The figure shows three views and two pictorial views of one solid part (mm, origin at its lowest corner). Answer the questions. A direction names the side the tool comes from. Round coordinates to 2 decimals unless told otherwise and drop trailing zeros. Order: outer loops, then holes, each group sorted by start corner. A loop starts at its lowest first (then second) coordinate and runs counter-clockwise, first axis right, second up. Notation, with made-up numbers: M 14.25,85.5 L 21.25,85.5 A23 ccw 21.25,110.5 Z; hole C -2,39 d5. An arc over 180 degrees is marked long. Return JSON: item names as keys, results as strings.
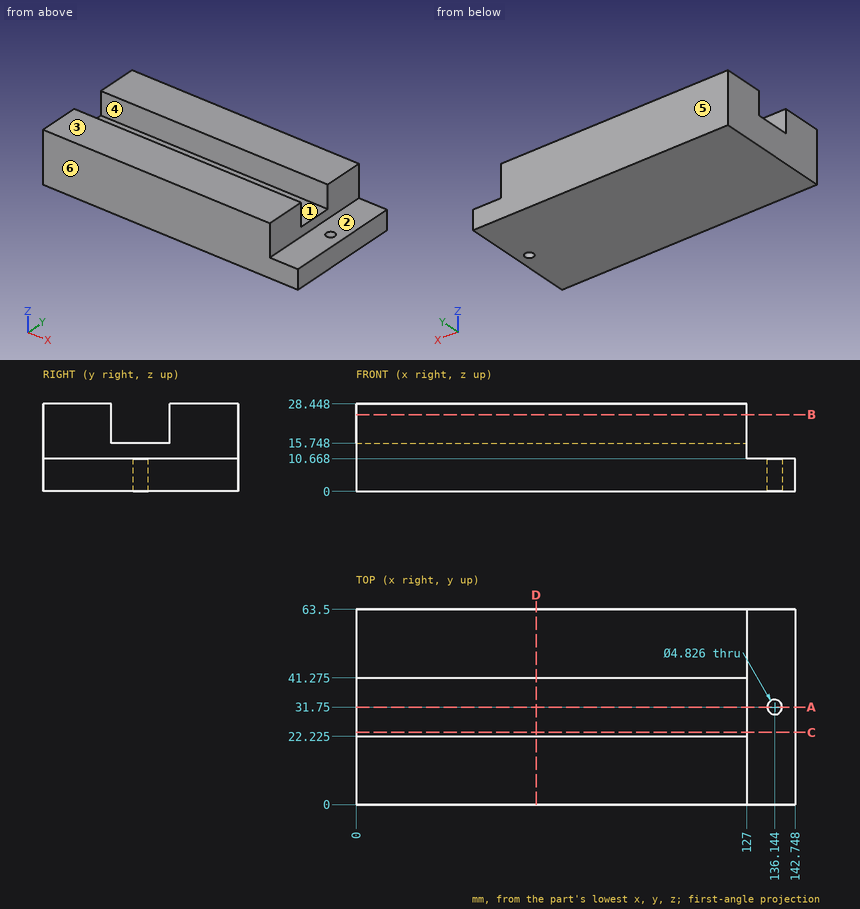
Item 1: Each of these flat-tipped pins is pushed along its axis until it touches: pin 1 (9.5 mm diameter, centred on x = 52, y = 35.5, fed in from +Z); pin 2 (8 mm diameter, centred on x = 135.5, y = 36.5, fed in from +Z); pin 3 (1.5 mm diameter, centred on y = 30, z = 17.5, fed in from +X). Where does it stop, or does it pass through?
Output:
{"pin 1": "stops at z = 15.75", "pin 2": "stops at z = 10.67", "pin 3": "passes through"}
Item 2: Find section B-B (z = 25). Determine the outline of the cut face in (x, y) (3 decimals).
Output:
{"outline": "M 0,0 L 127,0 L 127,22.225 L 0,22.225 Z; M 0,41.275 L 127,41.275 L 127,63.5 L 0,63.5 Z"}
Item 3: The mould has two halves that part along Y. Classify the marked faces 4, 5 and 6: pulls with the +Y half, pulls with the -Y half, needs draft (parallel to the pull), parting line crosses it, or undercut.
Output:
{"face 4": "undercut", "face 5": "pulls with the +Y half", "face 6": "pulls with the -Y half"}
Item 4: Find section A-A (y = 31.75). Determine the outline of the cut face in (x, z), plus the area to 3 significant figures.
Output:
{"outline": "M 0,0 L 133.73,0 L 133.73,10.67 L 127,10.67 L 127,15.75 L 0,15.75 Z; M 138.56,0 L 142.75,0 L 142.75,10.67 L 138.56,10.67 Z", "area": "2,120 mm^2"}
Item 5: Find section C-C (y = 23.5). Determine the outline of the cut face in (x, z).
Output:
{"outline": "M 0,0 L 142.75,0 L 142.75,10.67 L 127,10.67 L 127,15.75 L 0,15.75 Z"}
Item 6: Consider line 1 along Y through (x, z) = (113.5, 25.5) (3 decimals); line 2 along Z through (x, y) = (133, 29); line 3 along Z through (x, y) = (75.5, 41). Determine where each line is inside the solid, lowest interval first. Write a range as [from, to].
Output:
{"line 1": "y = [0, 22.225], [41.275, 63.5]", "line 2": "z = [0, 10.67]", "line 3": "z = [0, 15.75]"}
Item 7: Find section D-D (x = 58.5). Determine the outline of the cut face in (y, z) (3 decimals), plus the area to 3 significant figures.
Output:
{"outline": "M 0,0 L 63.5,0 L 63.5,28.448 L 41.275,28.448 L 41.275,15.748 L 22.225,15.748 L 22.225,28.448 L 0,28.448 Z", "area": "1,560 mm^2"}
Item 8: Which of the six approach directions +Z, -Z, +X, -X, +Y, -Y give full straight-line access (tool end or side, diameter ignored) to the marked faces 1, 2 and 3?
Output:
{"face 1": "+Z, +X, -X", "face 2": "+Z, +X, +Y, -Y", "face 3": "+Z, +X, -X, +Y, -Y"}
